Could you check a few things on this model? Use its own coordinates, in mm. Face numbers are marked on the shaded views. Give positions to 0.01 mm unless a question says otherwise; leave off trailing zeros. Order: outer loops, then holes, each group sorted by start corner. A loop starts at its lowest first (then second) coordinate and runs counter-clockwise, first axis right, second up. Notation, with made-up numbers: (15.5, 70.5) -> (55.5, 70.5) arc R13 cw to (55.5, 90.5) -> close; hole circle Ø4 at (-39.75, -6.75). An arc over 180 degrees is marked (long way). Write each question's results on one line, items separated by ' | '.
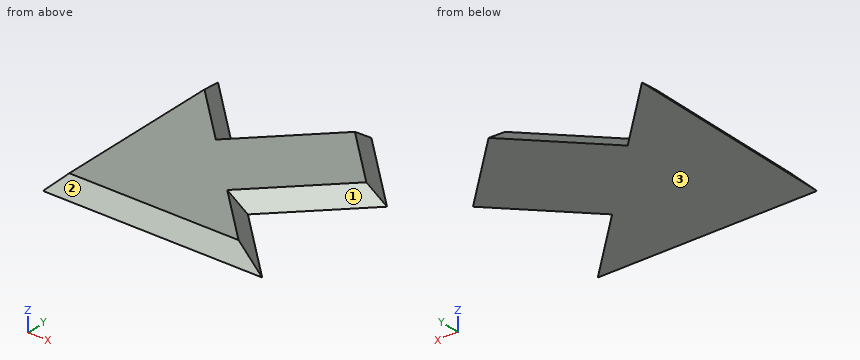
```python
from build123d import *

# Parameters (mm, degrees)
F1_DEPTH = 2
F2_SIZE  = 1.99999


# Not quite as in the source:
# - a fillet or chamfer is up to 0.001 mm smaller than in the source, because OpenCascade refuses the exact size


with BuildPart() as f1:
    # F0 (on Top) → F1 (new body)
    with BuildSketch(Plane.XY):
        Polygon((0, 30), (0, 0), (30, 0), (20.2933432917, 9.7066567083), (30.880029875, 20.2933432917), (20.2933432917, 30.880029875), (9.7066567083, 20.2933432917), align=None)
    extrude(amount=F1_DEPTH)

    # F2 (size 2 in the source; OpenCascade refuses exactly that, so slightly less here)
    f2_edges = [f1.edges().sort_by_distance(p)[0] for p in [
        (25.586687, 15, 2),
        (15, 25.586687, 2),
        (25.146672, 4.853328, 2),
        (15, 0, 2),
        (0, 15, 2),
        (4.853328, 25.146672, 2),
        (25.586687, 25.586687, 2),
    ]]
    chamfer(f2_edges, length=F2_SIZE)


solid = f1.part
```
Q1. Thinking about a two-plate mould opening in Y: for the marked faces 1, 2 and 3, which applies, +Y half, -Y half, draft (parallel to the pull), parting line (faces both ways), or undercut?
Here are the results:
face 1: undercut | face 2: -Y half | face 3: draft
Q2. I need wall thicknesses on line 1 along X through (y, z) = (21, 0.3); line 2 along Y through (x, z) = (21, 1.35); line 3 along Y through (x, z) = (24, 1.9). Which ranges of each line are inside material? Lowest first, please.
Here are the results:
line 1: x = 0.3 to 8.58, 10.84 to 29.75 | line 2: y = 1.35 to 7.09, 12.32 to 28.26 | line 3: y = 1.9 to 3.31, 16.1 to 24.49
Q3. I'm going to push a flat-ended pin straight in: pin 1 Ø3 at (x, y) = (27.5, 17) entering from +Z. Where does the tip first touch, or does it pass through?
Here are the results:
pin 1: stops at z = 1.56
Q4. Suppose I cut it at B-B on z = 0.55. Please give me the cut outline in (x, y), and give its area (3 significant figures).
Here are the results:
outline: (0.55, 0.55) -> (28.67, 0.55) -> (19.52, 9.71) -> (30.1, 20.29) -> (20.29, 30.1) -> (9.71, 19.52) -> (0.55, 28.67) -> close | area: 603 mm²
